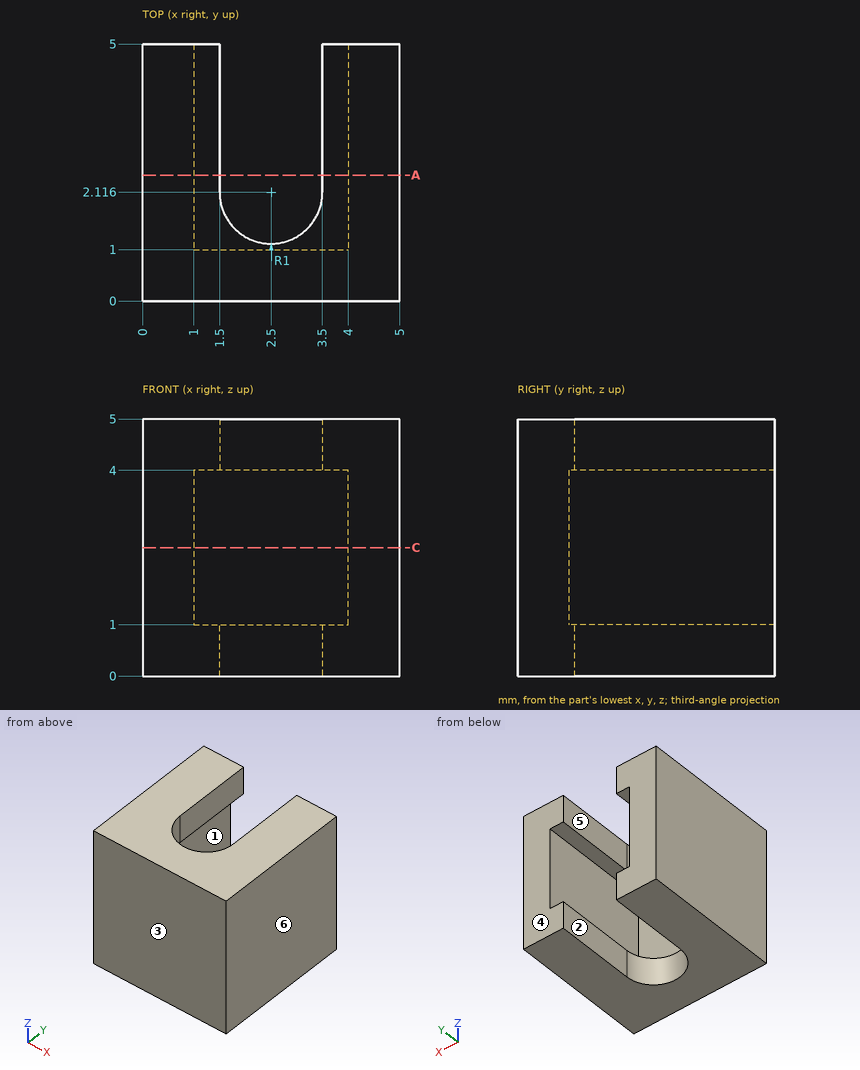
Design review of the part shown in the three views and the two pictorial views. Dimensions are in mm from the part's minimum x, y and z. A direction names the side the tool comes from. Round coordinates to 2 decimals unless told otherwise and drop trailing zeros. Write each loop counter-clockwise with the first axis right and the second up, starting at its lowest first coordinate (ties: lowest second). Pieces come first, ordered by that corner, then holes.
Item 1: Draft analysis for pull direction X (two halves, no side actions). For the marked faces 4, 5 and 6, state which applies: released by +X, released by -X, zero draft, split by the parting line, or undercut.
Item 2: Consider section A-A on y = 2.45. Give the boundary of the cut face in (x, z).
Item 3: For the marked faces 1, 2 and 3, list the 3-axis set-ups (+Z, -Z, +X, -X, +Y, -Y) from which the entire face can be reached by the end or side of a thin tool; tool diameter is ignored.
Item 4: Consider section C-C on z = 2.5. Give the boundary of the cut face in (x, y).
Item 5: Wall thickness on L1, parallel to X at y = 1.7, z = 3.1; L2, parallel to Y at x = 3.9, z = 2.95: over which ranges is each line inside the solid? List them lowest first.
Item 6: For pin 1 Ø1.5 at (x, z) = (3, 3) entering from +Y, flat-tipped, find the tip position at first contact; note if it passes through.
Check values:
1. face 4: zero draft
1. face 5: undercut
1. face 6: released by +X
2. outline: (0, 0) - (1.5, 0) - (1.5, 1) - (1, 1) - (1, 4) - (1.5, 4) - (1.5, 5) - (0, 5) - close; (3.5, 0) - (5, 0) - (5, 5) - (3.5, 5) - (3.5, 4) - (4, 4) - (4, 1) - (3.5, 1) - close
3. face 1: +Y
3. face 2: +Z, -Z, +Y
3. face 3: +Z, -Z, +X, -X, -Y
4. outline: (0, 0) - (5, 0) - (5, 5) - (4, 5) - (4, 1) - (1, 1) - (1, 5) - (0, 5) - close
5. L1: x = 0 to 1, 4 to 5
5. L2: y = 0 to 1
6. pin 1: stops at y = 1
